For this review, take the finished solid that the model builds, in its own axes (mm). A direction names the side the tool comes from. Round coordinates to 2 decimals unless told otherwise and drop trailing zeros. Write each loop counter-clockwise with the first axis right and the second up, starting at its lowest first coordinate (ties: lowest second). Pieces come first, ordered by that corner, then holes. Notation, with made-up numbers: (66, -18) - (104, -18) arc R20 cw to (104, 5) - close; hole circle Ø3 at (-15.5, 76). An arc over 180 degrees is marked (long way). One line per item, written item: value. Start each with the question number.
Q1. For probe 1 along X at (y, z) = (1.25, 0); probe 2 along X at (y, z) = (-1, 0); probe 3 along Y at (x, z) = (15, -13), list the stretches that pass through material, from the lowest coordinate up.
Q2. Mouldability with a two-part tool opening along X and no side actions: class faces 1 (the face through (0.3, -2, 5.3)), 2 (the face through (3.69, 8, 0)), 3 (the face through (19.372, -0.986, -4.835)), 4 (the face through (22.5, -1, -0.1)) as +X half, -X half, draft (parallel to the pull), parting line (faces both ways), or undercut.
Q3. Add section A-A on x = 0. Write out the cut boundary in (y, z).
Q4. Add section C-C on y = 8. Write out the cut boundary in (x, z), and give its area (3 significant figures).
Q5. Tool access review of faces 5 (the face through (-9.7, 4.9, -12.6)), 6 (the face through (0, 10, -4)), 7 (the face through (19.372, -0.986, 4.835)): name each direction out of +Z, -Z, +X, -X, +Y, -Y from which nothing blocks a thin tool from reaching the whole face with its end or side.
Q6. Add section B-B on z = 0. Write out the cut boundary in (x, y).
Q7. Add section D-D on y = 3.75. Write out the cut boundary in (x, z).
Q8. Clearance check with flat-ended pins moving along their axes: pin 1 Ø7.5 at (x, z) = (0, 0) entering from -Y; pin 2 Ø2.5 at (x, z) = (0, 12.5) entering from +Y; pin 3 Ø1.1 at (x, y) = (-0.5, 7.5) entering from +Z. State where each tip first meets the part, or that it passes through.
```python
from build123d import *

# Parameters (mm, degrees)
SKETCH_1_R          = 15.9
EXTRUDE_1_DEPTH     = 10
SKETCH_2_R          = 22.5
EXTRUDE_2_DEPTH     = 2
SKETCH_3_R          = 1.5
CUT_EXTRUDE_3_DEPTH = 3
CUT_EXTRUDE_4_DEPTH = 3
CUT_EXTRUDE_5_DEPTH = 5
CUT_EXTRUDE_START   = -7
SKETCH_6_R          = 4.15
CUT_EXTRUDE_6_DEPTH = 7
CHAMFER_1_SIZE      = 1


with BuildPart() as part:
    # Эскиз1 → Вытянуть1 (new body)
    with BuildSketch(Plane(origin=(0, 0, 0), x_dir=(1, 0, 0), z_dir=(0, 1, 0))):
        with Locations(Location((0, 0, 0), (0, 0, 270))):
            Circle(SKETCH_1_R)
    extrude(amount=EXTRUDE_1_DEPTH)

    # Эскиз2 → Вытянуть2 (add)
    with BuildSketch(Plane.XZ):
        with Locations(Location((0, 0, 0), (0, 0, 270))):
            Circle(SKETCH_2_R)
    extrude(amount=EXTRUDE_2_DEPTH)

    # Эскиз3 → Вытянуть3 (cut)
    with BuildSketch(Plane(origin=(0, 10, 0), x_dir=(1, 0, 0), z_dir=(0, 1, 0))):
        with Locations(Location((0, 12.5, 0), (0, 0, 270))):
            Circle(SKETCH_3_R)
        with Locations(Location((0, -12.5, 0), (0, 0, 270))):
            Circle(SKETCH_3_R)
    extrude(amount=-CUT_EXTRUDE_3_DEPTH, mode=Mode.SUBTRACT)

    # Эскиз4 → Вытянуть4 (cut)
    with BuildSketch(Plane(origin=(0, 0, 0), x_dir=(1, 0, 0), z_dir=(0, 1, 0))):
        with BuildLine():
            Line((21.764513428, 5.705782614), (16.912221051, 3.939692621))
            Line((16.912221051, 3.939692621), (17.254241194, 3))
            Line((17.254241194, 3), (21.997944585, 4.726566834))
            ThreePointArc((21.997944585, 4.726566834), (21.886705981, 5.217480357), (21.764513428, 5.705782614))
        make_face()
        with BuildLine():
            Line((17.254241194, -3), (21.997944585, -4.726566834))
            ThreePointArc((21.997944585, -4.726566834), (21.886705981, -5.217480357), (21.764513428, -5.705782614))
            Line((21.764513428, -5.705782614), (16.912221051, -3.939692621))
            Line((16.912221051, -3.939692621), (17.254241194, -3))
        make_face()
    extrude(amount=-CUT_EXTRUDE_4_DEPTH, mode=Mode.SUBTRACT)

    # Эскиз5 → Вытянуть5 (cut)
    with BuildSketch(Plane(origin=(0, 10, 0), x_dir=(1, 0, 0), z_dir=(0, 1, 0))):
        with BuildLine():
            Line((3.689512163, 1.9), (3.689512163, -1.9))
            ThreePointArc((3.689512163, -1.9), (-2.934493142, -2.934493142), (-1.9, 3.689512163))
            Line((-1.9, 3.689512163), (1.9, 3.689512163))
            ThreePointArc((1.9, 3.689512163), (2.934493142, 2.934493142), (3.689512163, 1.9))
        make_face()
    extrude(amount=-CUT_EXTRUDE_5_DEPTH, mode=Mode.SUBTRACT)

    # Эскиз6 → Вытянуть6 (cut)
    with BuildSketch(Plane.XZ.offset(2).offset(CUT_EXTRUDE_START)):
        with Locations(Location((0, 0, 0), (0, 0, 27.247255186))):
            Circle(SKETCH_6_R)
    extrude(amount=CUT_EXTRUDE_6_DEPTH, mode=Mode.SUBTRACT)

    # Фаска1
    chamfer_1_edges = [part.edges().sort_by_distance(p)[0] for p in [
        (-3.689512163, -2, -1.9),
    ]]
    chamfer(chamfer_1_edges, length=CHAMFER_1_SIZE)


solid = part.part
```
Result set:
1. probe 1: x = -15.9 to -4.15, 4.15 to 15.9
1. probe 2: x = -22.5 to -4.15, 4.15 to 22.5
1. probe 3: y = -2 to 0
2. face 1: draft
2. face 2: undercut
2. face 3: undercut
2. face 4: +X half
3. outline: (-2, -22.5) - (0, -22.5) - (0, -15.9) - (10, -15.9) - (10, -14) - (7, -14) - (7, -11) - (10, -11) - (10, -3.69) - (5, -3.69) - (5, -4.15) - (-1, -4.15) - (-2, -5.15) - close; (-2, 5.15) - (-1, 4.15) - (10, 4.15) - (10, 11) - (7, 11) - (7, 14) - (10, 14) - (10, 15.9) - (0, 15.9) - (0, 22.5) - (-2, 22.5) - close
4. outline: circle Ø31.8 at (0, 0); hole (-1.9, -3.69) - (1.9, -3.69) arc R4.15 ccw to (3.69, -1.9) - (3.69, 1.9) arc R4.15 ccw (long way) to start; hole circle Ø3 at (0, -12.5); hole circle Ø3 at (0, 12.5)
4. area: 728 mm^2
5. face 5: +Y
5. face 6: +Z, -Z, +X, -X, +Y
5. face 7: +Y, -Y
6. outline: (-22.5, -2) - (-5.15, -2) - (-4.15, -1) - (-4.15, 10) - (-15.9, 10) - (-15.9, 0) - (-22.5, 0) - close; (3.69, 5) - (4.15, 5) - (4.15, -1) - (5.15, -2) - (22.5, -2) - (22.5, 0) - (15.9, 0) - (15.9, 10) - (3.69, 10) - close
7. outline: circle Ø31.8 at (0, 0); hole circle Ø8.3 at (0, 0)
8. pin 1: stops at y = 5
8. pin 2: stops at y = 7
8. pin 3: stops at z = 15.9
